The figure shows three views and two pictorial views of one solid part (mm, origin at its lowest corner). Answer the questions. A direction names the side the tool comes from. Coordinates: 2 decimals unless noted, no trailing zeros. Loops run counter-clockwise (first coordinate to the right, second up) from the corner with the lowest first, then second, coordinate; pieces in that order, holes last. Notation, with made-up numbers: (-5, -39.5) -> (18, -39.5) arc R19 cw to (18, -16.5) -> close; hole circle Ø3 at (16.5, 40). An arc over 180 degrees is marked (long way). Answer in a Markdown table with one row per item.
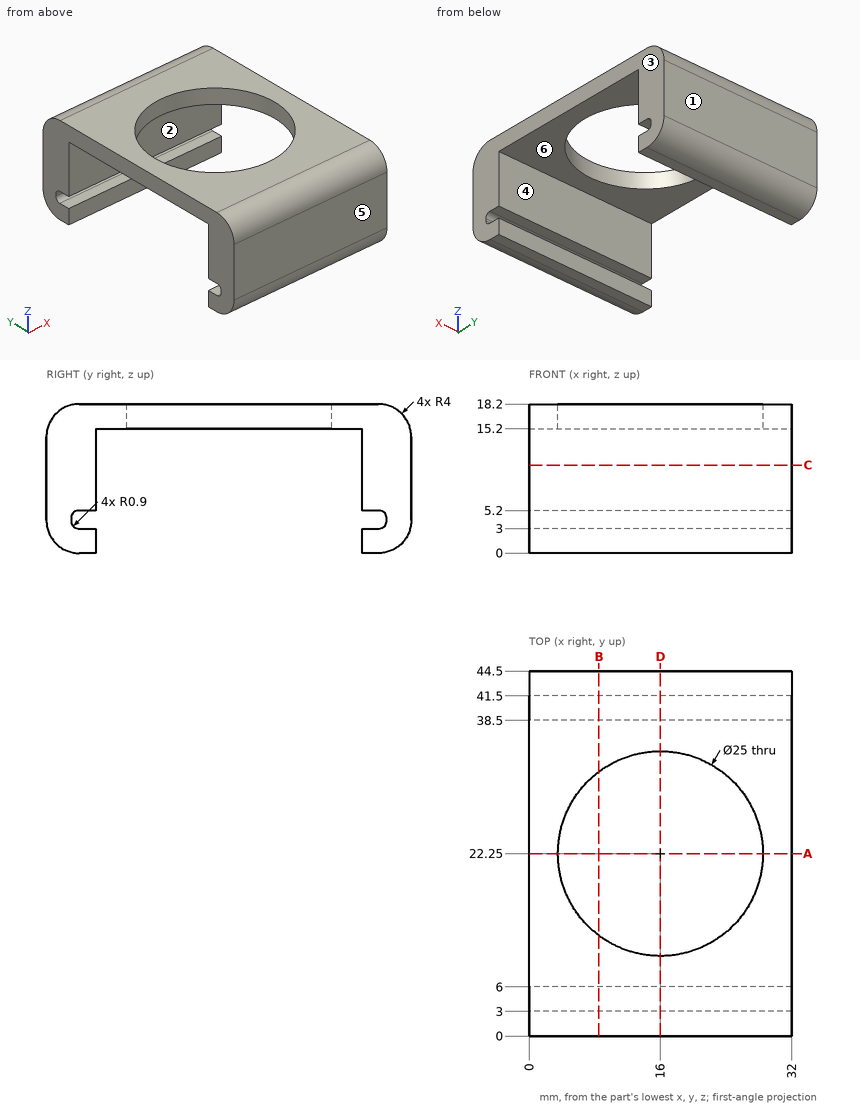
Item 1: Flat-ended cylindrical pins translate along their axes: pin 1 Ø1 at (x, y) = (22, 5) entering from -Z; pin 2 Ø16 at (x, y) = (11, 19.5) entering from -Z; pin 3 Ø2 at (y, z) = (20, 12.5) entering from -X; pin 4 Ø2.5 at (x, z) = (15, 2) entering from +Y. Find the tip coordinate at first contact, or state that the pin passes through.
Findings below:
| item | result |
|---|---|
| pin 1 | stops at z = 0 |
| pin 2 | stops at z = 15.2 |
| pin 3 | passes through |
| pin 4 | stops at y = 44.43 |
Item 2: Determine the mould class of the marked faces 3, 4, 5 and 6 for opening direction Y: +Y half, -Y half, draft (parallel to the pull), parting line (faces both ways), or undercut.
Findings below:
| item | result |
|---|---|
| face 3 | draft |
| face 4 | undercut |
| face 5 | -Y half |
| face 6 | undercut |
Item 3: A tool of negligible diameter and unlimited length cuts with its end or side. For the marked faces 1 and 2, from which of +Z, -Z, +X, -X, +Y, -Y can it reach the whole face along a straight path? Write none if from no direction.
Findings below:
| item | result |
|---|---|
| face 1 | +Z, -Z, +X, -X, +Y |
| face 2 | -Z, +X, -X |
Item 4: A cutting plane is placed at B-B, the plane x = 8.5. Determine the outline of the cut face in (y, z).
Findings below:
| item | result |
|---|---|
| outline | (0, 4) arc R4 ccw to (4, 0) -> (6, 0) -> (6, 3) -> (3.9, 3) arc R0.9 cw to (3, 3.9) -> (3, 4.3) arc R0.9 cw to (3.9, 5.2) -> (6, 5.2) -> (6, 15.2) -> (12.25, 15.2) -> (12.25, 18.2) -> (4, 18.2) arc R4 ccw to (0, 14.2) -> close; (32.25, 15.2) -> (38.5, 15.2) -> (38.5, 5.2) -> (40.6, 5.2) arc R0.9 cw to (41.5, 4.3) -> (41.5, 3.9) arc R0.9 cw to (40.6, 3) -> (38.5, 3) -> (38.5, 0) -> (40.5, 0) arc R4 ccw to (44.5, 4) -> (44.5, 14.2) arc R4 ccw to (40.5, 18.2) -> (32.25, 18.2) -> close |
Item 5: A cutting plane is placed at D-D, the plane x = 16. Determine the outline of the cut face in (y, z), plus the area to 3 significant figures.
Findings below:
| item | result |
|---|---|
| outline | (0, 4) arc R4 ccw to (4, 0) -> (6, 0) -> (6, 3) -> (3.9, 3) arc R0.9 cw to (3, 3.9) -> (3, 4.3) arc R0.9 cw to (3.9, 5.2) -> (6, 5.2) -> (6, 15.2) -> (9.75, 15.2) -> (9.75, 18.2) -> (4, 18.2) arc R4 ccw to (0, 14.2) -> close; (34.75, 15.2) -> (38.5, 15.2) -> (38.5, 5.2) -> (40.6, 5.2) arc R0.9 cw to (41.5, 4.3) -> (41.5, 3.9) arc R0.9 cw to (40.6, 3) -> (38.5, 3) -> (38.5, 0) -> (40.5, 0) arc R4 ccw to (44.5, 4) -> (44.5, 14.2) arc R4 ccw to (40.5, 18.2) -> (34.75, 18.2) -> close |
| area | 215 mm2 |
Item 6: A cutting plane is placed at C-C, the plane z = 10.75. Determine the outline of the cut face in (x, y), plus the area to 3 significant figures.
Findings below:
| item | result |
|---|---|
| outline | (0, 0) -> (32, 0) -> (32, 6) -> (0, 6) -> close; (0, 38.5) -> (32, 38.5) -> (32, 44.5) -> (0, 44.5) -> close |
| area | 384 mm2 |
Item 7: Find the intervals of material crossed by probe 1 along Y at (x, z) = (5, 10.25); probe 2 along Z at (x, y) = (25, 40.5); probe 3 along Y at (x, z) = (20.5, 4.25), in increasing order.
Findings below:
| item | result |
|---|---|
| probe 1 | y = 0 to 6, 38.5 to 44.5 |
| probe 2 | z = 0 to 3, 5.2 to 18.2 |
| probe 3 | y = 0 to 3, 41.5 to 44.5 |
Item 8: A cutting plane is placed at A-A, the plane y = 22.25. Determine the outline of the cut face in (x, z).
Findings below:
| item | result |
|---|---|
| outline | (0, 15.2) -> (3.5, 15.2) -> (3.5, 18.2) -> (0, 18.2) -> close; (28.5, 15.2) -> (32, 15.2) -> (32, 18.2) -> (28.5, 18.2) -> close |
